Build history of the part. All positions in model axes, mm. Face numbers are marked on the shaded views. A direction names the side the tool comes from. Coordinates: 2 decimals unless noted, no trailing zeros. Write each loop counter-clockwise with the first axis right and the second up, starting at its lowest first coordinate (ties: lowest second). Pieces come first, ordered by that corner, then holes.
```python
from build123d import *

# Parameters (mm, degrees)
EXTRUDE_1_DEPTH        = 6
HOLE_WIZARD_M6_2_D     = 5
HOLE_WIZARD_M6_2_DEPTH = 15
HOLE_WIZARD_M6_2_TIP   = 1.502151548
HOLE_WIZARD_M6_1_D     = 5
HOLE_WIZARD_M6_1_DEPTH = 15
HOLE_WIZARD_M6_1_TIP   = 1.502151548


with BuildPart() as part:
    # 草图1 → 凸台-拉伸1 (new, symmetric)
    with BuildSketch(Plane(origin=(0, 0, 0), x_dir=(1, 0, 0), z_dir=(0, 1, 0))):
        Polygon((0, 0), (25, 0), (25, -45), (15, -45), (0, -10), align=None)
    extrude(amount=EXTRUDE_1_DEPTH, both=True)

    # M6 螺纹孔2
    with Locations(Plane(origin=(25, 0, 0), x_dir=(0, 0, -1), z_dir=(1, 0, 0))):
        with Locations((-20, 0), (-40, 0)):
            Hole(HOLE_WIZARD_M6_2_D / 2, depth=HOLE_WIZARD_M6_2_DEPTH)
            with Locations((0, 0, -(HOLE_WIZARD_M6_2_DEPTH + HOLE_WIZARD_M6_2_TIP / 2))):  # 118° drill point
                Cone(0, HOLE_WIZARD_M6_2_D / 2, HOLE_WIZARD_M6_2_TIP, mode=Mode.SUBTRACT)

    # M6 螺纹孔1
    with Locations(Plane(origin=(0, 0, 0), x_dir=(-1, 0, 0), z_dir=(0, 0, -1))):
        with Locations((-6, 0)):
            Hole(HOLE_WIZARD_M6_1_D / 2, depth=HOLE_WIZARD_M6_1_DEPTH)
            with Locations((0, 0, -(HOLE_WIZARD_M6_1_DEPTH + HOLE_WIZARD_M6_1_TIP / 2))):  # 118° drill point
                Cone(0, HOLE_WIZARD_M6_1_D / 2, HOLE_WIZARD_M6_1_TIP, mode=Mode.SUBTRACT)


solid = part.part
```
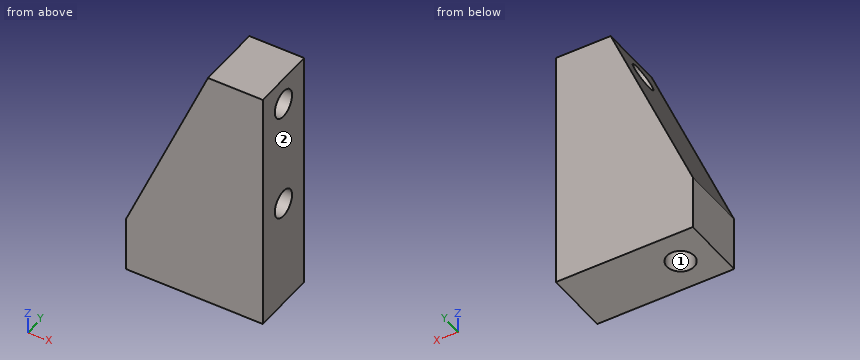
1. Probe line 1 along Z through (x, y) = (17.5, 0); line 2 along Y through (x, z) = (20.75, 40); line 3 along X through (y, z) = (0, 9). List the from-to ranges inside material, lowest first.
Computed values:
line 1: z = 0 to 17.5, 22.5 to 37.5, 42.5 to 45
line 2: y = -6 to -2.5, 2.5 to 6
line 3: x = 0 to 3.5, 8.5 to 25
2. Saw through at C-C on z = 6.5. List the corners of the cut face in (x, y), plus the area to 3 significant figures.
Computed values:
outline: (0, -6) - (25, -6) - (25, 6) - (0, 6) - close; hole circle Ø5 at (6, 0)
area: 280 mm2
3. Saw through at D-D on y = 4.75. List the corners of the cut face in (x, z), plus the area to 4 significant figures.
Computed values:
outline: (0, 0) - (25, 0) - (25, 45) - (15, 45) - (0, 10) - close
area: 862.5 mm2
4. 3-axis set-ups, long thin cutter, end or side, ignore diameter. For the marked faces 1 and 2: which of +Z, -Z, +X, -X, +Y, -Y reach the whole face in a straight line?
Computed values:
face 1: -Z
face 2: +Z, -Z, +X, +Y, -Y
5. Saw through at A-A on x = 21.25. List the corners of the cut face in (y, z), plus the area to 3 significant figures.
Computed values:
outline: (-6, 0) - (6, 0) - (6, 45) - (-6, 45) - close; hole circle Ø5 at (0, 20); hole circle Ø5 at (0, 40)
area: 501 mm2
6. Saw through at B-B on z = 39. List the corners of the cut face in (x, y), plus the area to 3 significant figures.
Computed values:
outline: (12.43, -6) - (25, -6) - (25, -2.29) - (12.43, -2.29) - close; (12.43, 2.29) - (25, 2.29) - (25, 6) - (12.43, 6) - close
area: 93.2 mm2
7. Flat gauge pins, fed straight in: pin 1 (5 mm diameter, centred on y = -0.5, z = 40, fed in from -X); pin 2 (4.5 mm diameter, centred on y = 0, z = 40, fed in from +X); pin 3 (6 mm diameter, centred on y = 0, z = 20, fed in from -X). Where does each tip first touch, or does it go through?
Computed values:
pin 1: stops at x = 11.79
pin 2: passes through
pin 3: stops at x = 3
